from build123d import *

# Parameters (mm, degrees)
SKETCH1_W           = 40
SKETCH1_H           = 40
SKETCH1_R           = 1
BOSS_EXTRUDE1_DEPTH = 0.8
SKETCH4_W           = 4.6
SKETCH4_H           = 12
BOSS_EXTRUDE2_DEPTH = 12.8
SKETCH5_R           = 0.6
CUT_EXTRUDE1_DEPTH  = 6
CUT_EXTRUDE2_DEPTH  = 6


with BuildPart() as part:
    # Sketch1 → Boss-Extrude1 (new body)
    with BuildSketch(Plane.XY):
        with Locations((0.062552029, -0.069037071)):
            Rectangle(SKETCH1_W, SKETCH1_H)
        with Locations((17.862552029, -17.869037071)):
            Circle(SKETCH1_R, mode=Mode.SUBTRACT)
        with Locations((17.862552029, 17.730962929)):
            Circle(SKETCH1_R, mode=Mode.SUBTRACT)
        with Locations((-17.737447971, 17.730962929)):
            Circle(SKETCH1_R, mode=Mode.SUBTRACT)
        with Locations((-17.737447971, -17.869037071)):
            Circle(SKETCH1_R, mode=Mode.SUBTRACT)
    extrude(amount=BOSS_EXTRUDE1_DEPTH)

    # Sketch4 → Boss-Extrude2 (add)
    with BuildSketch(Plane.XY.offset(0.8)):
        with Locations((12.562552029, -5.569037071)):
            Rectangle(SKETCH4_W, SKETCH4_H)
        with Locations((-15.437447971, -5.569037071)):
            Rectangle(SKETCH4_W, SKETCH4_H)
    extrude(amount=-BOSS_EXTRUDE2_DEPTH)

    # Sketch5 → Cut-Extrude1 (cut)
    with BuildSketch(Plane(origin=(0, 0.430962929, 0), x_dir=(1, 0, 0), z_dir=(0, 1, 0))):
        with Locations(Location((-15.437447971, 6.2, 0), (0, 0, 180))):
            Circle(SKETCH5_R)
        with Locations(Location((12.562552029, 6.2, 0), (0, 0, 180))):
            Circle(SKETCH5_R)
    extrude(amount=-CUT_EXTRUDE1_DEPTH, mode=Mode.SUBTRACT)

    # Sketch6 → Cut-Extrude2 (cut)
    with BuildSketch(Plane(origin=(0, 0, 0), x_dir=(-1, 0, 0), z_dir=(0, 0, -1))):
        with BuildLine():
            Line((7.737447971, 10.930962929), (-13.262552029, 10.930962929))
            ThreePointArc((-13.262552029, 10.930962929), (-15.762552029, 13.430962929), (-13.262552029, 15.930962929))
            Line((-13.262552029, 15.930962929), (7.737447971, 15.930962929))
            ThreePointArc((7.737447971, 15.930962929), (10.237447971, 13.430962929), (7.737447971, 10.930962929))
        make_face()
    extrude(amount=-CUT_EXTRUDE2_DEPTH, mode=Mode.SUBTRACT)


solid = part.part
Here's how the part is built. I have some questions about the finished solid (model axes, mm). A direction names the side the tool comes from. Round coordinates to 2 decimals unless told otherwise and drop trailing zeros. Loops run counter-clockwise (first coordinate to the right, second up) from the corner with the lowest first, then second, coordinate; pieces in that order, holes last.
1. If we section it at D-D on z = -6.2: Write out the boundary of the cut face in (x, y), plus the area to 3 significant figures.
Answer list:
outline: (-17.74, -11.57) - (-13.14, -11.57) - (-13.14, 0.43) - (-14.84, 0.43) - (-14.84, -5.57) - (-16.04, -5.57) - (-16.04, 0.43) - (-17.74, 0.43) - close; (10.26, -11.57) - (14.86, -11.57) - (14.86, 0.43) - (13.16, 0.43) - (13.16, -5.57) - (11.96, -5.57) - (11.96, 0.43) - (10.26, 0.43) - close
area: 96.0 mm2
2. If we section it at C-C on y = -9: Write out the boundary of the cut face in (x, z), plus the area to 3 significant figures.
Answer list:
outline: (-19.94, 0) - (-17.74, 0) - (-17.74, -12) - (-13.14, -12) - (-13.14, 0) - (10.26, 0) - (10.26, -12) - (14.86, -12) - (14.86, 0) - (20.06, 0) - (20.06, 0.8) - (-19.94, 0.8) - close
area: 142 mm2
3. If I drill on line 1 along X through (y, z) = (-2, -0.5); line 2 along Z through (x, y) = (-4.5, -18); line 3 along Y through (x, z) = (-14.5, -8.25), over which ranges is the centre line in solid material (lowest first)?
Answer list:
line 1: x = -17.74 to -13.14, 10.26 to 14.86
line 2: z = 0 to 0.8
line 3: y = -11.57 to 0.43
4. For P1, Ø3, axis at x = -6, y = -6.5, coming from the -Z side; P2, Ø5, axis at x = 12, z = -4, coming from the -Y side; P3, Ø1.4, axis at x = 12.56, z = -6.2, coming from the +Y side, each with a flat end and sliding along its axis, tell me the tip position at first contact or that it passes through.
Answer list:
P1: stops at z = 0
P2: stops at y = -11.57
P3: stops at y = 0.43
5. If we section it at B-B on x = 0: Write out the boundary of the cut face in (y, z), plus the area to 3 significant figures.
Answer list:
outline: (-20.07, 0) - (10.93, 0) - (10.93, 0.8) - (-20.07, 0.8) - close; (15.93, 0) - (19.93, 0) - (19.93, 0.8) - (15.93, 0.8) - close
area: 28.0 mm2
6. Which directions (+Z, -Z, +X, -X, +Y, -Y) give clear straight access to the entire face, cutting with the end or side of a thin tool? Please do faces 1 (the face through (13.16, -2.53, -6.17)), 2 (the face through (-15, -11.569, -6)), 3 (the face through (10.263, -6, -6)), 4 (the face through (11.5, 0.431, -5.9)).
Answer list:
face 1: +Y
face 2: -Z, +X, -X, -Y
face 3: -Z, +Y, -Y
face 4: -Z, +X, -X, +Y
7. We'd pull the mould along X, two halves only. Please class faces 5 (the face through (17.07, 17.12, 0.39)), 6 (the face through (-17.737, -6, -6)), 7 (the face through (13, -11.569, -6)): +X half, -X half, draft (parallel to the pull), parting line (faces both ways), or undercut.
Answer list:
face 5: undercut
face 6: -X half
face 7: draft
8. If we section it at A-A on z = -2: Write out the boundary of the cut face in (x, y).
Answer list:
outline: (-17.74, -11.57) - (-13.14, -11.57) - (-13.14, 0.43) - (-17.74, 0.43) - close; (10.26, -11.57) - (14.86, -11.57) - (14.86, 0.43) - (10.26, 0.43) - close
